from build123d import *

# Parameters (mm, degrees)
CUT_EXTRUDE1_DEPTH      = 4.318
SKETCH4_W               = 6.35
SKETCH4_H               = 3.3274
CUT_EXTRUDE2_DEPTH      = 7.112
CUT_EXTRUDE3_DEPTH      = 22.07205187
CUT_EXTRUDE3_DEPTH_BACK = 22.07205187
SKETCH5_R               = 0.79375
FILLET2_R               = 1.27


with BuildPart() as part:
    # Sketch2 → Revolve1 (revolve)
    with BuildSketch(Plane.XY, mode=Mode.PRIVATE) as revolve1_sk:
        Polygon((9.525, 0), (9.525, 5.08), (5.08, 5.08), (5.08, 11.176), (0, 11.176), (0, 0), align=None)
    revolve(revolve1_sk.sketch.rotate(Axis((0, 11.176, 0), (0, -1, 0)), 180), axis=Axis((0, 11.176, 0), (0, -1, 0)))

    # Sketch3 → Cut-Extrude1 (cut)
    with BuildSketch(Plane.XZ):
        Polygon((6.452466608, 0), (3.226233304, 5.588), (-3.226233304, 5.588), (-6.452466608, 0), (-3.226233304, -5.588), (3.226233304, -5.588), align=None)
    extrude(amount=-CUT_EXTRUDE1_DEPTH, mode=Mode.SUBTRACT)

    # Sketch4 → Cut-Extrude2 (cut)
    with BuildSketch(Plane(origin=(0, 11.176, 0), x_dir=(1, 0, 0), z_dir=(0, 1, 0))):
        Rectangle(SKETCH4_W, SKETCH4_H)
    extrude(amount=-CUT_EXTRUDE2_DEPTH, mode=Mode.SUBTRACT)

    # Sketch5 → Cut-Extrude3 (cut, two sides: drawn at the far end of the back side and taken through both)
    with BuildSketch(Plane.XY.offset(-5.588).offset(-CUT_EXTRUDE3_DEPTH_BACK)):
        with Locations((0, 2.159)):
            Circle(SKETCH5_R)
    extrude(amount=CUT_EXTRUDE3_DEPTH + CUT_EXTRUDE3_DEPTH_BACK, mode=Mode.SUBTRACT)

    # Fillet2
    fillet2_edges = [part.edges().sort_by_distance(p)[0] for p in [
        (9.525, 5.08, 0),
    ]]
    fillet(fillet2_edges, radius=FILLET2_R)


solid = part.part
Work out the finished part from the listing and answer in its coordinate system (mm). A direction names the side the tool comes from. Give positions to 0.01 mm unless a question says otherwise; leave off trailing zeros. Loops run counter-clockwise (first coordinate to the right, second up) from the corner with the lowest first, then second, coordinate; pieces in that order, holes last. Notation, with made-up numbers: (36, -5.5) - (93, -5.5) arc R12 cw to (93, 4.5) - close; hole circle Ø7 at (48, 51). An arc over 180 degrees is marked (long way). Answer in a Markdown table with one row per item.
(1) Section B-B (y = 7) is taken. Give the vertices of the cut face in (x, z) (3 decimals).
Results list:
| item | result |
|---|---|
| outline | circle Ø10.16 at (0, 0); hole (-3.175, -1.664) - (3.175, -1.664) - (3.175, 1.664) - (-3.175, 1.664) - close |
(2) Flat-ended cylindrical pins translate along their axes: pin 1 Ø6 at (x, z) = (6.5, -3) entering from -Y; pin 2 Ø1.3 at (x, y) = (1, 2.5) entering from +Z; pin 3 Ø4 at (y, z) = (10, -2.5) entering from +X; pin 4 Ø1.7 at (y, z) = (7, -0.5) entering from -X. Find the tip coordinate at first contact, or state that the pin passes through.
Results list:
| item | result |
|---|---|
| pin 1 | stops at y = 0 |
| pin 2 | stops at z = 9.52 |
| pin 3 | stops at x = 5.06 |
| pin 4 | stops at x = -5.08 |
(3) Consider L1, parallel to Y at x = 0, z = -6.4; L2, parallel to Z at x = 0, y = 3 (3 decimals); L3, parallel to Z at x = -2.25, y = 7. Determine where each line is inside the solid, lowest interval first. Write a range as [from, to].
Results list:
| item | result |
|---|---|
| L1 | y = [0, 1.37], [2.95, 5.08] |
| L2 | z = [-9.525, -5.588], [5.588, 9.525] |
| L3 | z = [-4.55, -1.66], [1.66, 4.55] |
(4) Section A-A (x = 0) is taken. Give the vertices of the cut face in (y, z) (3 decimals).
Results list:
| item | result |
|---|---|
| outline | (0, -9.525) - (1.365, -9.525) - (1.365, -5.588) - (0, -5.588) - close; (0, 5.588) - (1.365, 5.588) - (1.365, 9.525) - (0, 9.525) - close; (2.953, -9.525) - (3.81, -9.525) arc R1.27 ccw to (5.08, -8.255) - (5.08, -5.08) - (11.176, -5.08) - (11.176, -1.664) - (4.318, -1.664) - (4.318, -5.588) - (2.953, -5.588) - close; (2.953, 5.588) - (4.318, 5.588) - (4.318, 1.664) - (11.176, 1.664) - (11.176, 5.08) - (5.08, 5.08) - (5.08, 8.255) arc R1.27 ccw to (3.81, 9.525) - (2.953, 9.525) - close |
(5) A tool of negligible diameter and unlimited length cuts with its end or side. For faces 1 (the face through (0, 11.176, 2)), 2 (the face through (0, 4.318, -2)), 3 (the face through (0, 8, 1.664)), from which of +Z, -Z, +X, -X, +Y, -Y can it reach the whole face along a straight path? Write none if from no direction.
Results list:
| item | result |
|---|---|
| face 1 | +Z, -Z, +X, -X, +Y |
| face 2 | -Y |
| face 3 | +Y, -Y |
(6) For a pull along X with two mould halves and no side action, classify faces 4 (the face through (4, 5.08, 4)), 5 (the face through (-1, 2, 5.588)), 6 (the face through (0.661, 8.171, -5.037)) as pulls with the +X half, pulls with the -X half, needs draft (parallel to the pull), parting line crosses it, or undercut.
Results list:
| item | result |
|---|---|
| face 4 | needs draft |
| face 5 | undercut |
| face 6 | parting line crosses it |
